For this review, take the finished solid that the model builds, in its own axes (mm). A direction names the side the tool comes from. Coordinates: 2 decimals unless noted, no trailing zeros. Write each loop counter-clockwise with the first axis right and the second up, starting at its lowest first coordinate (ties: lowest second). Pieces come first, ordered by that corner, then holes. Notation, with made-up numbers: (-2.5, -12.75) - (1.5, -12.75) arc R14 ccw to (1.5, -5.75) - close; hole circle Ø6 at (89.5, 51.5). An arc over 180 degrees is marked (long way). Write each question's results on one line, items separated by ' | '.
Autodesk Inventor part; units mm, degrees
ref_plane "YZ Plane" through (0, 0, 0) normal (1, 0, 0) x (0, 1, 0)
ref_plane "XZ Plane" through (0, 0, 0) normal (0, 1, 0) x (-1, 0, 0)
ref_plane "XY Plane" through (0, 0, 0) normal (0, 0, 1) x (1, 0, 0)
sketch "Sketch1" plane through (0, 0, 0) normal (0, 0, 1) x (1, 0, 0)
  line L0 (0, 0) -> (104.775, 0)
  line L1 (104.775, 0) -> (104.775, 137.16)
  line L2 (104.775, 137.16) -> (0, 137.16)
  line L3 (0, 137.16) -> (0, 0)
  dimension "d0" = 104.775
  dimension "d1" = 137.16
extrude "Extrusion1" add sketch "Sketch1" along normal blind 9.525
sketch "Sketch2" plane through (0, 0, 9.525) normal (0, 0, 1) x (1, 0, 0)
  line L0 (0, 137.16) -> (104.775, 137.16)
  line L1 (0, 0) -> (9.525, 0)
  line L2 (9.525, 0) -> (9.525, 137.16)
  line L3 (9.525, 137.16) -> (0, 137.16)
  line L4 (0, 137.16) -> (0, 0)
  dimension "d4" = 9.525
extrude "Extrusion2" add sketch "Sketch2" along normal blind 406.4
properties part number "l_bracket" material "Aluminum-6061"
Q1. Take a section at B-B on x = 72. State the section outline as (y, z) points (3 decimals), plus the area to 3 significant figures.
Results found:
outline: (0, 0) - (137.16, 0) - (137.16, 9.525) - (0, 9.525) - close | area: 1,310 mm2
Q2. Take a section at A-A on y = 39. State the section outline as (x, z) points (3 decimals), plus the area to 3 significant figures.
Results found:
outline: (0, 0) - (104.775, 0) - (104.775, 9.525) - (9.525, 9.525) - (9.525, 415.925) - (0, 415.925) - close | area: 4,870 mm2
Q3. Take a section at C-C on z = 109. State the section outline as (x, y) points (3 decimals), plus the area to 3 significant figures.
Results found:
outline: (0, 0) - (9.525, 0) - (9.525, 137.16) - (0, 137.16) - close | area: 1,310 mm2
Q4. Wall thickness on line 1 along X through (y, z) = (77, 22.5) (3 decimals): over which ranges is the line inside the solid? List them lowest first. Write a range as from..to.
Results found:
line 1: 0..9.525
Q5. For pin 1 (12 mm diameter, centred on x = 44.5, y = 91, fed in from +Z) (3 decimals); pin 2 (3 mm diameter, centred on x = 37.5, y = 108, fed in from -Z); pin 3 (12 mm diameter, centred on y = 102, z = 74, fed in from +X) (3 decimals), all flat-tipped, find the tip position at first contact; note any pin that passes through.
Results found:
pin 1: z = 9.525 | pin 2: z = 0 | pin 3: x = 9.525
Q6. For faces 1 (the face through (9.525, 68, 210)), 2 (the face through (52, 70, 0)), list the 3-axis set-ups (+Z, -Z, +X, -X, +Y, -Y) from which the entire face can be reached by the end or side of a thin tool; tool diameter is ignored.
Results found:
face 1: +Z, +X, +Y, -Y | face 2: -Z, +X, -X, +Y, -Y
